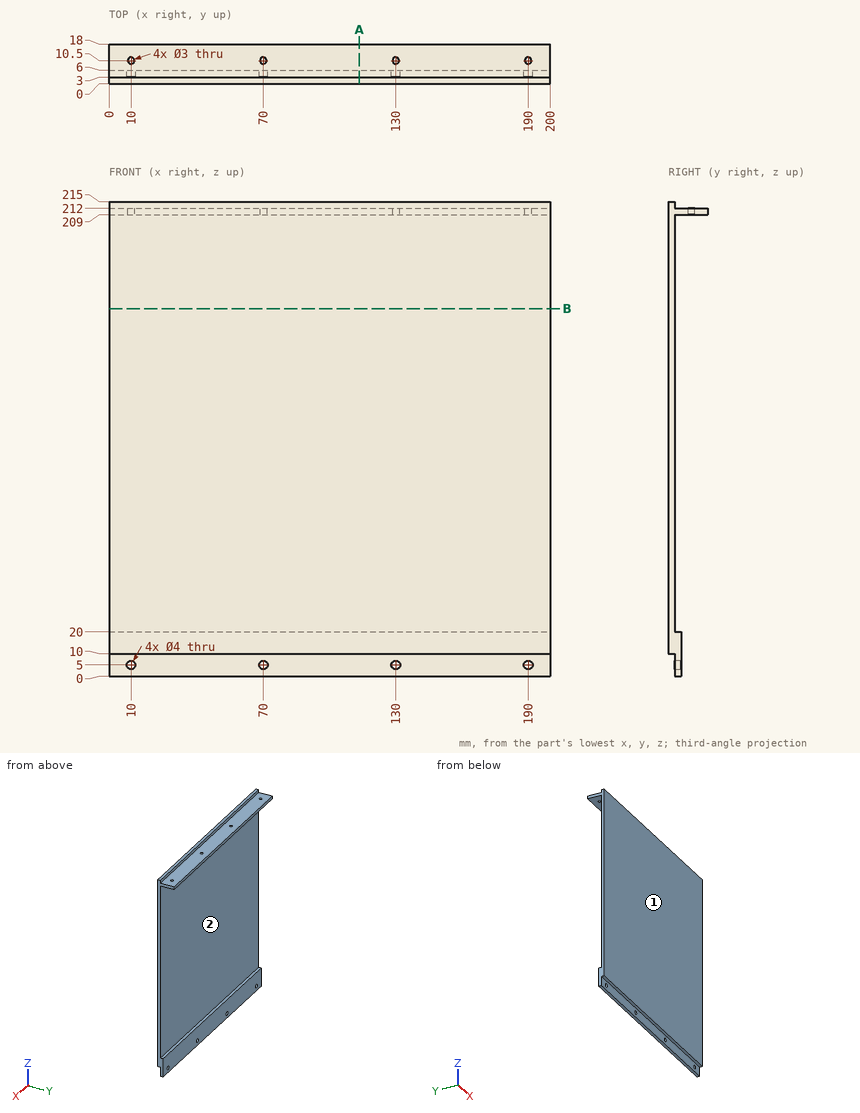
Geometry: see drawing. Coordinates: mm, zero at the bounding-box minimum. Give positions to 0.01 mm unless a question says otherwise; leave off trailing zeros. Order: outer loops, then holes, each group sorted by start corner. A loop starts at its lowest first (then second) coordinate and runs counter-clockwise, first axis right, second up. Notation, with made-up numbers: (-11, -9) -> (4, -9) arc R36 cw to (4, 28) -> close; hole circle Ø1 at (-36, 62). An arc over 180 degrees is marked (long way). Write each question's results on one line, items separated by ' | '. Start each with the question number.
1) Section B-B (z = 166.5). Return loops of the section in (x, y), then the cut area to 3 significant figures.
2) Draft query along Z for the marked faces 1 and 2. Return one class per face: pulls with the +Z half, pulls with the -Z half, needs draft (parallel to the pull), parting line crosses it, or undercut.
3) First-contact query: pin 1 (1.5 mm diameter, centred on x = 87.5, y = 1, fed in from -Z); pin 2 (3 mm diameter, centred on x = 85.5, z = 3, fed in from -Y); pin 3 (4 mm diameter, centred on x = 10, y = 10.5, fed in from -Z). Flat tips, straight axial feed; report the tip coordinate or a pass-through.
4) Section A-A (x = 113.5). Return loops of the section in (y, z), then the cut area to 3 significant figures.
5) Line query: line 1 (X direction, y = 5.35, z = 5); line 2 (Z direction, x = 70, y = 3.95); line 3 (Y direction, x = 10, z = 209.95). Output: solid intervals per line, ascending. Write a range as from..to.
Calculated:
1) outline: (0, 0) -> (200, 0) -> (200, 3) -> (0, 3) -> close | area: 600 mm2
2) face 1: needs draft | face 2: undercut
3) pin 1: z = 10 | pin 2: y = 3 | pin 3: z = 209
4) outline: (0, 10) -> (3, 10) -> (3, 0) -> (6, 0) -> (6, 20) -> (3, 20) -> (3, 209) -> (18, 209) -> (18, 212) -> (3, 212) -> (3, 215) -> (0, 215) -> close | area: 720 mm2
5) line 1: 0..8, 12..68, 72..128, 132..188, 192..200 | line 2: 0..3, 7..20, 209..212 | line 3: 0..9, 12..18
